Build history of the part. All positions in model axes, mm. Face numbers are marked on the shaded views. A direction names the side the tool comes from. Give positions to 0.01 mm unless a question says otherwise; leave off trailing zeros. Order: outer loops, then holes, each group sorted by start corner. A loop starts at its lowest first (then second) coordinate and runs counter-clockwise, first axis right, second up. Notation, with made-up numbers: (-27.75, -39.75) -> (25.25, -39.75) arc R9 ccw to (25.25, -26.75) -> close; hole circle Ø3 at (73.5, 52). An arc over 180 degrees is marked (long way). One line per item, written item: value. Start each with the question number.
(1) Which spindle directions (+Z, -Z, +X, -X, +Y, -Y) get a long thin tool onto all of the face, cutting with end or side? Do the marked faces 1, 2 and 3. Say none if no direction does.
(2) Probe line 1 (Z direction, x = 6, y = 0); line 2 (Y direction, x = 3.5, z = 0); line 3 (Y direction, x = 12.55, z = 0). List the from-to ranges inside material, lowest first.
(3) Saw through at A-A on x = 3.5. Give the cut face in (y, z), plus the area to 3 significant figures.
(4) Pin check, flat tips, straight feed: pin 1 (3 mm diameter, centred on x = 6.5, z = -2.5, fed in from -Y); pin 2 (1.2 mm diameter, centred on y = 5, z = -1, fed in from +X); pin 3 (2.5 mm diameter, centred on x = 9.5, z = 1.5, fed in from +Y); pin 4 (2.5 mm diameter, centred on y = 0, z = -2, fed in from +X). Stop position of each tip, or through.
(5) Two-plate mould, pull along Y, no slides. Class the marked faces 4, 5 and 6: +Y half, -Y half, draft (parallel to the pull), parting line (faces both ways), or undercut.
```python
from build123d import *

# Parameters (mm, degrees)
SKETCH2_W          = 0.381
SKETCH2_H          = 3.9624
SKETCH4_W          = 49.3268
SKETCH4_H          = 24.6634
SKETCH4_W_2        = 24.6634
SKETCH4_H_2        = 9.398
CUT_EXTRUDE1_DEPTH = 4.7752


with BuildPart() as part:
    # Sketch1 → Revolve1 (revolve)
    with BuildSketch(Plane.XY):
        Polygon((0, 0), (0, 4.90855), (0.762, 5.67055), (3.7592, 5.67055), (4.2672, 5.16255), (4.7752, 5.16255), (4.7752, 6.16585), (11.938, 6.16585), (12.7, 5.40385), (12.7, 0), align=None)
    revolve(axis=Axis((12.7, 0, 0), (-1, 0, 0)))

    # Sketch2 → Cut-Revolve1 (revolve, cut)
    with BuildSketch(Plane.XY):
        with Locations((12.5095, 1.9812)):
            Rectangle(SKETCH2_W, SKETCH2_H)
    revolve(axis=Axis((12.7, 0, 0), (-1, 0, 0)), mode=Mode.SUBTRACT)

    # Sketch3 → Cut-Revolve2 (revolve, cut)
    with BuildSketch(Plane.XY):
        Polygon((0, 0), (0, 1.98374), (11.88974, 1.98374), (12.319, 2.413), (12.319, 0), align=None)
    revolve(axis=Axis((12.319, 0, 0), (-1, 0, 0)), mode=Mode.SUBTRACT)

    # Sketch4 → Cut-Extrude1 (cut)
    with BuildSketch(Plane(origin=(12.7, 0, 0), x_dir=(0, 0, -1), z_dir=(1, 0, 0))):
        Rectangle(SKETCH4_W, SKETCH4_H)
        Rectangle(SKETCH4_W_2, SKETCH4_H_2, mode=Mode.SUBTRACT)
    extrude(amount=-CUT_EXTRUDE1_DEPTH, mode=Mode.SUBTRACT)

    # Sketch5 → Revolve2 (revolve)
    with BuildSketch(Plane.XY):
        with BuildLine():
            Line((4.066488686, 6.16585), (4.066488686, 6.081681804))
            Line((4.066488686, 6.081681804), (4.663607684, 5.484562806))
            ThreePointArc((4.663607684, 5.484562806), (4.700805122, 5.394760245), (4.663607684, 5.304957684))
            Line((4.663607684, 5.304957684), (4.5212, 5.16255))
            Line((4.5212, 5.16255), (4.2672, 5.16255))
            Line((4.2672, 5.16255), (4.2672, 4.90855))
            Line((4.2672, 4.90855), (4.7752, 4.90855))
            Line((4.7752, 4.90855), (4.7752, 5.660338686))
            Line((4.7752, 5.660338686), (4.269688686, 6.16585))
            Line((4.269688686, 6.16585), (4.066488686, 6.16585))
        make_face()
    revolve(axis=Axis((4.7752, 0, 0), (-1, 0, 0)))


solid = part.part
```
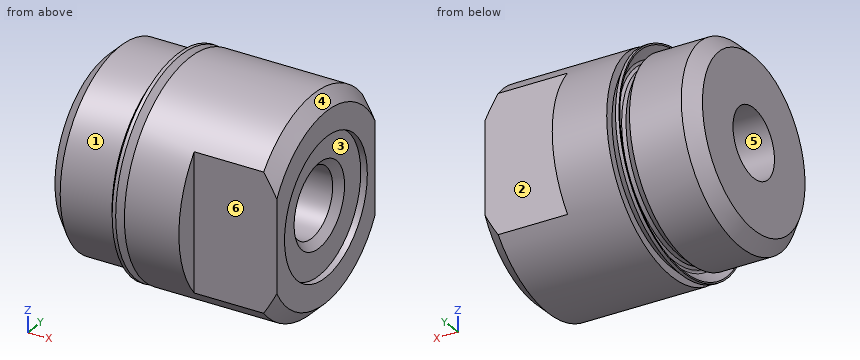
Results below:
1. face 1: -X
1. face 2: +Z, -Z, +X, +Y
1. face 3: +X
2. line 1: z = -6.17 to -1.98, 1.98 to 6.17
2. line 2: y = -5.67 to -1.98, 1.98 to 5.67
2. line 3: y = -4.7 to -3.96, 3.96 to 4.7
3. outline: circle Ø11.34 at (0, 0); hole circle Ø3.97 at (0, 0)
3. area: 88.7 mm²
4. pin 1: stops at y = -6.08
4. pin 2: stops at x = 12.7
4. pin 3: stops at y = 4.7
4. pin 4: stops at x = 12.32
5. face 4: parting line
5. face 5: undercut
5. face 6: -Y half
